Verification items for the finished model (mm, model axes). Face numbers are marked on the shaded views. A direction names the side the tool comes from. Round coordinates to 2 decimals unless told otherwise and drop trailing zeros. Write each loop counter-clockwise with the first axis right and the second up, starting at its lowest first coordinate (ties: lowest second). Pieces come first, ordered by that corner, then holes.
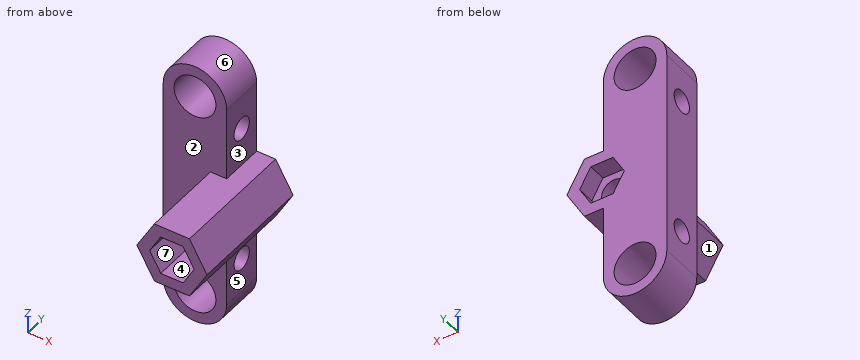
from build123d import *

# Parameters (mm, degrees)
SKETCH1_R           = 7.5875
BOSS_EXTRUDE1_DEPTH = 16
SKETCH2_R           = 4.0875
CUT_EXTRUDE1_DEPTH  = 63.988598267
SKETCH1_6_R         = 4.5
BOSS_EXTRUDE2_DEPTH = 9.5
BOSS_EXTRUDE3_DEPTH = 30


with BuildPart() as part:
    # Sketch1 → Boss-Extrude1 (new body)
    with BuildSketch(Plane(origin=(0, 0, 0), x_dir=(1, 0, 0), z_dir=(0, 1, 0))):
        with BuildLine():
            Line((-23.5, -33), (-23.5, 33))
            Line((-23.5, 33), (-23.5, 37.5))
            ThreePointArc((-23.5, 37.5), (-12, 49), (-0.5, 37.5))
            Line((-0.5, 37.5), (-0.5, 33))
            Line((-0.5, 33), (-0.5, 11))
            Line((-0.5, 11), (6.350852961, 11))
            Line((6.350852961, 11), (12.701705922, 0))
            Line((12.701705922, 0), (6.350852961, -11))
            Line((6.350852961, -11), (-0.5, -11))
            Line((-0.5, -11), (-0.5, -33))
            Line((-0.5, -33), (-0.5, -37.5))
            ThreePointArc((-0.5, -37.5), (-12, -49), (-23.5, -37.5))
            Line((-23.5, -37.5), (-23.5, -33))
        make_face()
        with Locations(Location((-12, -37.5, 0), (0, 0, 270))):
            Circle(SKETCH1_R, mode=Mode.SUBTRACT)
        with Locations(Location((-12, 37.5, 0), (0, 0, 270))):
            Circle(SKETCH1_R, mode=Mode.SUBTRACT)
        Polygon((8.082903769, 0), (4.041451884, 7), (-4.041451884, 7), (-8.082903769, 0), (-4.041451884, -7), (4.041451884, -7), align=None, mode=Mode.SUBTRACT)
    extrude(amount=BOSS_EXTRUDE1_DEPTH)

    # Sketch2 → Cut-Extrude1 (cut, through all)
    with BuildSketch(Plane.ZY.offset(23.5)):
        with Locations((-25, 8)):
            Circle(SKETCH2_R)
        with Locations((25, 8)):
            Circle(SKETCH2_R)
    extrude(amount=-CUT_EXTRUDE1_DEPTH, mode=Mode.SUBTRACT)

    # Sketch1<6> → Boss-Extrude2 (add)
    with BuildSketch(Plane(origin=(0, 0, 0), x_dir=(1, 0, 0), z_dir=(0, 1, 0))):
        Polygon((-4.041451884, -7), (4.041451884, -7), (8.082903769, 0), (4.041451884, 7), (-4.041451884, 7), (-8.082903769, 0), align=None)
        with Locations(Location((0, 0, 0), (0, 0, 270))):
            Circle(SKETCH1_6_R, mode=Mode.SUBTRACT)
    extrude(amount=BOSS_EXTRUDE2_DEPTH)

    # Sketch4 → Boss-Extrude3 (add)
    with BuildSketch(Plane.XZ):
        Polygon((12.701705922, 0), (6.350852961, 11), (-6.350852961, 11), (-12.701705922, 0), (-6.350852961, -11), (6.350852961, -11), align=None)
        Polygon((8.082903769, 0), (4.041451884, 7), (-4.041451884, 7), (-8.082903769, 0), (-4.041451884, -7), (4.041451884, -7), align=None, mode=Mode.SUBTRACT)
    extrude(amount=BOSS_EXTRUDE3_DEPTH)


solid = part.part
Q1. Release check for a two-part mould opening along Z. For the marked faces 5, 6 and 7 record: released by +Z, released by -Z, zero draft, split by the parting line, or undercut.
Recorded:
face 5: zero draft
face 6: released by +Z
face 7: undercut
Q2. Sectioned sample at C-C (x = -2.5). Enter the section's corners in (y, z) (1 decimal).
Recorded:
outline: (-30, -11) - (0, -11) - (0, -44) - (16, -44) - (16, -7) - (9.5, -7) - (9.5, -3.7) - (0, -3.7) - (0, -7) - (-30, -7) - close; (-30, 7) - (0, 7) - (0, 3.7) - (9.5, 3.7) - (9.5, 7) - (16, 7) - (16, 44) - (0, 44) - (0, 11) - (-30, 11) - close; hole circle Ø8.2 at (8, -25); hole circle Ø8.2 at (8, 25)
Q3. Sectioned sample at B-B (z = 25). Enter the section's corners in (x, y).
Recorded:
outline: (-23.5, 0) - (-0.5, 0) - (-0.5, 3.91) - (-23.5, 3.91) - close; (-23.5, 12.09) - (-0.5, 12.09) - (-0.5, 16) - (-23.5, 16) - close
Q4. Tool access check on the marked faces 1, 2, 3 and 4. Record the directions out of +Z, -Z, +X, -X, +Y, -Y that give a thin tool (end or side, any length) a straight path to the whole face; none if there is none.
Recorded:
face 1: -Z, -X, -Y
face 2: -X, -Y
face 3: +Z, +X, +Y, -Y
face 4: -Y
Q5. Depth check by flat-ended pin: P1, Ø3, axis at x = -13, y = -10.5, coming from the +Z side; P2, Ø4, axis at x = -19, z = -6, coming from the -Y side; P3, Ø10, axis at x = -0.5, y = -8, coming from the +Z side. Enter the tip coordinate at first touch or a pass-through.
Recorded:
P1: stops at z = 2.08
P2: stops at y = 0
P3: stops at z = 11
Q6. Material ranges on line 1 along X through (y, z) = (2.5, 0); line 2 along X through (y, z) = (6, -37.5); line 3 along Z through (x, y) = (-1.5, -23.5), recorded low to high.
Recorded:
line 1: x = -23.5 to -4.5, 4.5 to 12.7
line 2: x = -23.5 to -19.59, -4.41 to -0.5
line 3: z = -11 to -7, 7 to 11
Q7. Sectioned sample at D-D (y = -23). Enter the section's corners in (x, z).
Recorded:
outline: (-12.7, 0) - (-6.35, -11) - (6.35, -11) - (12.7, 0) - (6.35, 11) - (-6.35, 11) - close; hole (-8.08, 0) - (-4.04, -7) - (4.04, -7) - (8.08, 0) - (4.04, 7) - (-4.04, 7) - close
Q8. Sectioned sample at A-A (y = 8). Enter the section's corners in (x, z) (1 decimal), plus the area to 3 significant figures.
Recorded:
outline: (-23.5, -37.5) arc R11.5 ccw to (-0.5, -37.5) - (-0.5, -29.1) - (-23.5, -29.1) - close; (-23.5, -20.9) - (-0.5, -20.9) - (-0.5, -11) - (6.4, -11) - (12.7, 0) - (6.4, 11) - (-0.5, 11) - (-0.5, 20.9) - (-23.5, 20.9) - close; (-23.5, 29.1) - (-0.5, 29.1) - (-0.5, 37.5) arc R11.5 ccw to (-23.5, 37.5) - close; hole circle Ø15.2 at (-12, -37.5); hole circle Ø15.2 at (-12, 37.5); hole circle Ø9 at (0, 0)
area: 1,560 mm2
